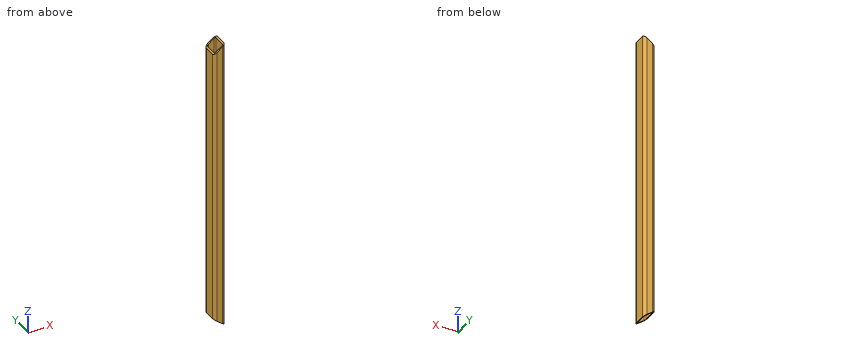
Autodesk Inventor part; units mm, degrees
ref_plane "Start Plane" through (0, 0, -50.8) normal (0, 0, 1) x (1, 0, 0)
ref_plane "End Plane" through (0, 0, 1270) normal (0, 0, 1) x (1, 0, 0)
ref_plane "Work Plane4" through (-15.24, 0, 1239.52) normal (-0.6, 0, 0.8) x (0.8, 0, 0.6)
ref_plane "Start Plane" through (0, 0, -50.8) normal (0, 0, 1) x (1, 0, 0)
ref_plane "End Plane" through (0, 0, 1270) normal (0, 0, 1) x (1, 0, 0)
sketch "Sketch" plane through (0, 0, 0) normal (0, 0, 1) x (1, 0, 0)
  line L0 (-25.4, -25.4) -> (-25.4, 25.4)
  line L1 (-12.7, 38.1) -> (12.7, 38.1)
  line L2 (25.4, 25.4) -> (25.4, -25.4)
  line L3 (12.7, -38.1) -> (-12.7, -38.1)
  arc A0 (-25.4, -25.4) -> (-12.7, -38.1) centre (-12.7, -25.4) ccw
  arc A1 (-12.7, 38.1) -> (-25.4, 25.4) centre (-12.7, 25.4) ccw
  arc A2 (25.4, 25.4) -> (12.7, 38.1) centre (12.7, 25.4) ccw
  arc A3 (12.7, -38.1) -> (25.4, -25.4) centre (12.7, -25.4) ccw
  arc A4 (-12.7, 31.75) -> (-19.05, 25.4) centre (-12.7, 25.4) ccw
  line L4 (-12.7, 31.75) -> (12.7, 31.75)
  arc A5 (19.05, 25.4) -> (12.7, 31.75) centre (12.7, 25.4) ccw
  line L5 (19.05, 25.4) -> (19.05, -25.4)
  arc A6 (12.7, -31.75) -> (19.05, -25.4) centre (12.7, -25.4) ccw
  line L6 (12.7, -31.75) -> (-12.7, -31.75)
  arc A7 (-19.05, -25.4) -> (-12.7, -31.75) centre (-12.7, -25.4) ccw
  line L7 (-19.05, -25.4) -> (-19.05, 25.4)
  line L8 (0, 57.0224) -> (0, -57.0224) construction
  line L9 (-39.2424, 0) -> (39.2424, 0) construction
  dimension "d10" = 76.2
  dimension "d11" = 50.8
  dimension "d12" = 6.35
  dimension "d15" = 38.1
  dimension "d16" = 25.4
  dimension "d17" = 12.7
extrude "Body" add sketch "Sketch" along normal up to surface (1320.8 mm away) from surface at -50.8
sketch "Sketch3" plane through (0, 0, 0) normal (0, 0, 1) x (1, 0, 0)
  line L0 (0, 0) -> (10, 0)
ref_plane "Work Plane3" through (0, 0, 0) normal (0, -1, 0) x (1, 0, 0)
ref_plane "Work Plane4" through (-15.24, 0, 1239.52) normal (-0.6, 0, 0.8) x (0.8, 0, 0.6)
split "Split1" plane through (-15.24, 0, 1239.52) removes the side toward (-0.6, 0, 0.8)
ref_plane "Work Plane5" through (-421.64, 0, 284.48) normal (-0.6, 0, -0.8) x (-0.8, 0, 0.6)
split "Split2" plane through (-421.64, 0, 284.48) removes the side toward (-0.6, 0, -0.8)
sketch "Sketch4" plane through (0, 0, 0) normal (0, -1, 0) x (1, 0, 0)
  line L0 (-2, -50.8) -> (12, -50.8)
  line L1 (-2, 1270) -> (12, 1270)
  dimension "d19" = 1320.8
equation "\"d10\" = G_H"
equation "\"d11\" = G_W"
equation "\"d12\" = G_T"
equation "\"d15\" = 0.5 * d10"
equation "\"d16\" = 0.5 * d11"
equation "\"d17\" = G_IR"
equation "\"d3\" = G_L"
equation "\"G_W\" = 50.8"
equation "\"G_H\" = 76.2"
equation "\"G_T\" = 6.35"
equation "\"G_IR\" = 12.7"
equation "\"G_L\" = d19"
equation "\"G_OFFSET_START\" = 50.8"
equation "\"G_OFFSET_END\" = 50.8"
equation "\"d13\" = -G_OFFSET_START"
equation "\"B_L\" = 1219.2"
properties part number "AISC - 3 x 2 x 1/4 - 52" material "Steel, Mild"
Here's how the part is built. I have some questions about the finished solid (model axes, mm). Round coordinates to 2 decimals unless told otherwise and drop trailing zeros. Loops run counter-clockwise (first coordinate to the right, second up) from the corner with the lowest first, then second, coordinate; pieces in that order, holes last. Notation, with made-up numbers: (74.25, 61) -> (85.25, 61) arc R35 cw to (85.25, 100) -> close; hole circle Ø9 at (52.5, 40.5). An arc over 180 degrees is marked (long way). Answer as CSV lines item,"result".
1. If I drill on L1, parallel to Y at x = 8, z = 774; L2, parallel to X at y = -10, z = 404; L3, parallel to X at y = -31, z = 402, over which ranges is the centre line in solid material (lowest first)?
Final values:
L1,"y = -38.1 to -31.75, 31.75 to 38.1"
L2,"x = -25.4 to -19.05, 19.05 to 25.4"
L3,"x = -24.1 to -15.69, 15.69 to 24.1"
2. If we section it at C-C on z = 35.5: Please give me the cut outline in (x, y).
Final values:
outline,"(-25.4, -25.4) arc R12.7 ccw to (-12.7, -38.1) -> (12.7, -38.1) arc R12.7 ccw to (25.4, -25.4) -> (25.4, 25.4) arc R12.7 ccw to (12.7, 38.1) -> (-12.7, 38.1) arc R12.7 ccw to (-25.4, 25.4) -> close; hole (-19.05, -25.4) arc R6.35 ccw to (-12.7, -31.75) -> (12.7, -31.75) arc R6.35 ccw to (19.05, -25.4) -> (19.05, 25.4) arc R6.35 ccw to (12.7, 31.75) -> (-12.7, 31.75) arc R6.35 ccw to (-19.05, 25.4) -> close"
3. For pin 1 (4 mm diameter, centred on x = -12.5, y = 30.5, fed in from -Z); pin 2 (1 mm diameter, centred on x = 18, y = -16.5, fed in from +Z); pin 3 (1 mm diameter, centred on x = 14.5, z = 690, fed in from +Y); pin 4 (5 mm diameter, centred on x = 17.5, y = 2, fed in from +Z), each with a flat end and sliding along its axis, tell me the tip position at first contact or that it passes through.
Final values:
pin 1,"stops at z = -23.55"
pin 2,"passes through"
pin 3,"stops at y = 38.03"
pin 4,"stops at z = 1265.95"
4. If we section it at B-B on y = 4: Please give me the cut outline in (x, z).
Final values:
outline,"(-25.4, -12.7) -> (-19.05, -17.46) -> (-19.05, 1236.66) -> (-25.4, 1231.9) -> close; (19.05, -46.04) -> (25.4, -50.8) -> (25.4, 1270) -> (19.05, 1265.24) -> close"
5. If we section it at A-A on x = 1: Please give me the cut outline in (y, z).
Final values:
outline,"(-38.1, -32.5) -> (-31.75, -32.5) -> (-31.75, 1251.7) -> (-38.1, 1251.7) -> close; (31.75, -32.5) -> (38.1, -32.5) -> (38.1, 1251.7) -> (31.75, 1251.7) -> close"
